Autodesk Inventor part; units mm, degrees
ref_plane "YZ Plane" through (0, 0, 0) normal (1, 0, 0) x (0, 1, 0)
ref_plane "XZ Plane" through (0, 0, 0) normal (0, 1, 0) x (-1, 0, 0)
ref_plane "XY Plane" through (0, 0, 0) normal (0, 0, 1) x (1, 0, 0)
sketch "Sketch10" plane through (0, 0, 0) normal (0, 0, 1) x (1, 0, 0)
  line L0 (0, 6.985) -> (-9.5327, 6.985)
  line L1 (0, 0) -> (-9.5327, 0)
  line L2 (-18.1754, 0) -> (-27.7081, 0)
  line L3 (-27.7081, 6.985) -> (-18.1754, 6.985)
  arc A0 (-9.5327, 6.985) -> (-18.1754, 6.985) centre (-13.8541, 3.4925) ccw
  arc A1 (-18.1754, 0) -> (-9.5327, 0) centre (-13.8541, 3.4925) ccw
  circle A2 centre (-13.8541, 3.4925) radius 3.9688
  line L4 (-26.4104, 1.5875) -> (-19.0735, 1.5875)
  line L5 (-19.0735, 5.3975) -> (-26.4104, 5.3975)
  line L6 (-8.6346, 1.5875) -> (-1.2978, 1.5875)
  line L7 (-1.2978, 5.3975) -> (-8.6346, 5.3975)
  arc A3 (-19.0735, 5.3975) -> (-19.0735, 1.5875) centre (-13.8541, 3.4925) ccw
  arc A4 (-8.6346, 1.5875) -> (-8.6346, 5.3975) centre (-13.8541, 3.4925) ccw
  arc A5 (-26.4104, 5.3975) -> (-26.4104, 1.5875) centre (-13.8541, 3.4925) ccw
  arc A6 (-27.7081, 6.985) -> (-27.7081, 0) centre (-13.8541, 3.4925) ccw
  arc A7 (-1.2978, 1.5875) -> (-1.2978, 5.3975) centre (-13.8541, 3.4925) ccw
  arc A8 (0, 0) -> (0, 6.985) centre (-13.8541, 3.4925) ccw
  dimension "d59" = 7.9375
  dimension "d152" = 1.5875
  dimension "d153" = 1.5875
  dimension "d158" = 3.81
  dimension "d168" = 12.7
  dimension "d169" = 12.7
  dimension "d170" = 1.5875
  dimension "d172" = 1.5875
extrude "Extrusion33" add sketch "Sketch10" along normal blind 14.6844
sketch "Sketch28" plane through (0, 0, 14.6844) normal (0, 0, 1) x (1, 0, 0)
  circle A0 centre (-13.8541, 3.4925) radius 3.9687
  arc A1 (-26.4104, 5.3975) -> (-26.4104, 1.5875) centre (-13.8541, 3.4925) ccw
  arc A2 (-28.014, 5.3975) -> (-28.014, 1.5875) centre (-13.8541, 3.4925) ccw
  arc A3 (-1.2978, 1.5875) -> (-1.2978, 5.3975) centre (-13.8541, 3.4925) ccw
  arc A4 (0.3059, 1.5875) -> (0.3059, 5.3975) centre (-13.8541, 3.4925) ccw
  line L0 (-28.014, 5.3975) -> (-26.4104, 5.3975)
  line L1 (-26.4104, 1.5875) -> (-28.014, 1.5875)
  line L2 (-1.2978, 5.3975) -> (0.3059, 5.3975)
  line L3 (0.3059, 1.5875) -> (-1.2978, 1.5875)
  line L4 (-26.4104, 5.3975) -> (-19.0735, 5.3975)
  line L5 (-19.0735, 1.5875) -> (-26.4104, 1.5875)
  arc A5 (-26.4104, 5.3975) -> (-26.4104, 1.5875) centre (-13.8541, 3.4925) ccw
  arc A6 (-27.7081, 6.985) -> (-27.7081, 0) centre (-13.8541, 3.4925) ccw
  arc A7 (-1.2978, 1.5875) -> (-1.2978, 5.3975) centre (-13.8541, 3.4925) ccw
  arc A8 (0, 0) -> (0, 6.985) centre (-13.8541, 3.4925) ccw
extrude "Extrusion35" cut sketch "Sketch28" against normal blind 3.175 contours A1 L1 A2 L0 | A3 L2 A4 L3
sketch "Sketch30" plane through (0, 0, 14.6844) normal (0, 0, 1) x (1, 0, 0)
  circle A0 centre (-13.8541, 3.4925) radius 3.9687
  circle A1 centre (-13.8541, 7.4612) radius 0.3969
  circle A2 centre (-15.3728, 7.1591) radius 0.3969
  circle A3 centre (-16.6604, 6.2988) radius 0.3969
  circle A4 centre (-17.5207, 5.0113) radius 0.3969
  circle A5 centre (-17.8228, 3.4925) radius 0.3969
  circle A6 centre (-17.5207, 1.9737) radius 0.3969
  circle A7 centre (-16.6604, 0.6862) radius 0.3969
  circle A8 centre (-15.3728, -0.1741) radius 0.3969
  circle A9 centre (-13.8541, -0.4763) radius 0.3969
  circle A10 centre (-12.3353, -0.1741) radius 0.3969
  circle A11 centre (-11.0477, 0.6862) radius 0.3969
  circle A12 centre (-10.1874, 1.9737) radius 0.3969
  circle A13 centre (-9.8853, 3.4925) radius 0.3969
  circle A14 centre (-10.1874, 5.0113) radius 0.3969
  circle A15 centre (-11.0477, 6.2988) radius 0.3969
  circle A16 centre (-12.3353, 7.1591) radius 0.3969
  point P0 (0, 0)
  dimension "d179" = 0.7937
  dimension "d182" = 360
fillet "Fillet6" radius 25.4 4 edges at (-9.5327, 6.985, 7.3422) (-18.1754, 6.985, 7.3422) (-9.5327, 0, 7.3422) (-18.1754, 0, 7.3422)
fillet "Fillet7" radius 3.175 4 edges at (0.1754, 6.1956, 14.6844) (0.1754, 0.7894, 14.6844) (-27.8835, 6.1956, 14.6844) (-27.8835, 0.7894, 14.6844)
extrude "Extrusion41" add sketch "Sketch30" against normal up to surface (14.6844 mm away) contours A0 A13 | A0 A13 | A14 A0 | A0 A14 | A12 A0 | A0 A12 | A15 A0 | A0 A15 | A11 A0 | A0 A11 | A16 A0 | A0 A16 | A10 A0 | A0 A10 | A1 A0 | A0 A1 | A9 A0 | A0 A9 | A2 A0 | A0 A2 | A8 A0 | A0 A8 | A3 A0 | A0 A3 | A7 A0 | A0 A7 | A4 A0 | A0 A4 | A6 A0 | A0 A6 | A5 A0 | A0 A5
sketch "Sketch33" plane through (0, 0, 14.6844) normal (0, 0, 1) x (1, 0, 0)
  line L0 (-19.4103, 3.8894) -> (-8.2978, 3.8894)
  line L1 (-8.2978, 3.8894) -> (-8.2978, 3.0956)
  line L2 (-8.2978, 3.0956) -> (-19.4103, 3.0956)
  line L3 (-19.4103, 3.0956) -> (-19.4103, 3.8894)
  arc A0 (-17.803, 3.0961) -> (-17.803, 3.8889) centre (-17.8228, 3.4925) ccw
  arc A1 (-8.6346, 1.5875) -> (-8.6346, 5.3975) centre (-13.8541, 3.4925) ccw
  arc A2 (-19.0735, 5.3975) -> (-19.0735, 1.5875) centre (-13.8541, 3.4925) ccw
  point P0 (0, 0)
extrude "Extrusion42" cut sketch "Sketch33" against normal through all
properties part number "extender-bracket"
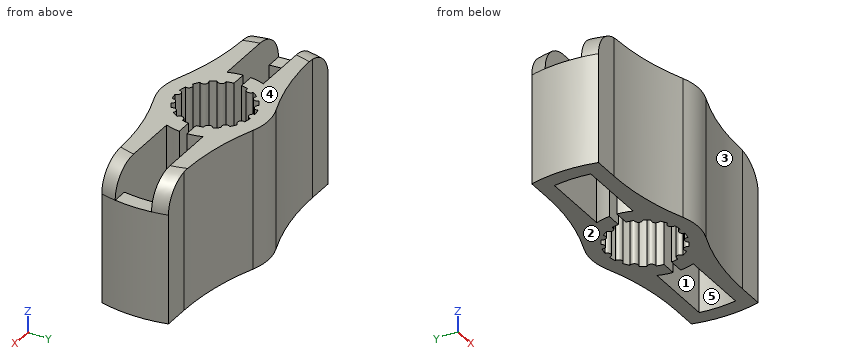
Read the model definition and answer for the solid it produces. Units are mm, in the model's axes. Face numbers are marked on the shaded views. A direction names the side the tool comes from. Give positions to 0.01 mm unless a question says otherwise; leave off trailing zeros. Write each loop counter-clockwise with the first axis right and the second up, starting at its lowest first coordinate (ties: lowest second). Pieces come first, ordered by that corner, then holes. Notation, with made-up numbers: M -2.75,-16.75 L 36.25,-16.75 A24 cw 36.25,17.25 Z; hole C 77,41.25 d7. An arc over 180 degrees is marked long. Put each result on its own line as item: value. Start each with the question number.
1. Which of the six approach directions +Z, -Z, +X, -X, +Y, -Y give full straight-line access (tool end or side, diameter ignored) to the marked faces 4 and 5?
2. The part is cut by section C-C, the plane y = -1.25. Give the vertices of the cut face in (x, z), and give its area (3 significant figures).
3. Each of these flat-tipped pins is pushed along its axis until it touches: pin 1 Ø2 at (x, z) = (-1, 7) entering from -Y; pin 2 Ø6 at (x, y) = (-9, -1) entering from +Z; pin 3 Ø5 at (x, z) = (-6, 4) entering from -Y; pin 4 Ø0.8 at (x, z) = (-9.5, 5) entering from -Y. Where does it stop, or does it pass through?
4. The part is cut by section A-A, the plane x = -21.5. Give the vertices of the cut face in (y, z).
5. Consider line 1 along Y through (x, z) = (-24.5, 2.75); line 2 along X through (y, z) = (3.25, 11.25); line 3 along Y through (x, z) = (-4.75, 4). Determine where each line is inside the solid, lowest interval first.
6. For a pull along X with two mould halves and no side action, classify the marked faces 1, 2 and 3 as released by +X, released by -X, zero draft, split by the parting line, or undercut.
7. The part is cut by section B-B, the plane x = -18.25. Give the vertices of the cut face in (y, z), and give its area (3 significant figures).
8. The part is cut by section D-D, the plane y = 7.75. Give the vertices of the cut face in (x, z), and give its area (3 significant figures).
Final values:
1. face 4: +Z, +X, -X, +Y, -Y
1. face 5: +Z, -Z
2. outline: M -17.1,0 L -10.61,0 L -10.61,14.68 L -17.1,14.68 Z
2. area: 95.3 mm²
3. pin 1: stops at y = 0
3. pin 2: stops at z = 14.68
3. pin 3: stops at y = -0.66
3. pin 4: stops at y = -1.03
4. outline: M -0.24,0 L 1.59,0 L 1.59,14.68 L -0.24,14.68 Z; M 5.4,0 L 7.22,0 L 7.22,14.68 L 5.4,14.68 Z
5. line 1: y = 0 to 1.59, 5.4 to 6.99
5. line 2: x = -28.14 to -26.55, -1.16 to 0.43
5. line 3: y = -0.08 to 1.59, 5.4 to 7.06
6. face 1: undercut
6. face 2: zero draft
6. face 3: released by +X
7. outline: M -0.9,0 L 3.1,0 L 3.1,14.68 L -0.9,14.68 Z; M 3.89,0 L 7.89,0 L 7.89,14.68 L 3.89,14.68 Z
7. area: 117 mm²
8. outline: M -18.78,0 L -8.93,0 L -8.93,14.68 L -18.78,14.68 Z
8. area: 145 mm²
